Autodesk Inventor part; units mm, degrees
ref_plane "YZ Plane" through (0, 0, 0) normal (1, 0, 0) x (0, 1, 0)
ref_plane "XZ Plane" through (0, 0, 0) normal (0, 1, 0) x (-1, 0, 0)
ref_plane "XY Plane" through (0, 0, 0) normal (0, 0, 1) x (1, 0, 0)
sketch "Sketch1" plane through (0, 0, 0) normal (0, 0, 1) x (1, 0, 0)
  circle A0 centre (0, 0) radius 4.05
  circle A1 centre (0, 0) radius 7.4
  line L0 (-8.7062, 0.25) -> (-2.7169, 0.25)
  line L1 (-2.7169, -0.25) -> (-8.7062, -0.25)
  line L2 (-8.7062, 0.25) -> (-8.7062, -0.25)
  line L3 (-2.7169, 0.25) -> (-2.7169, -0.25)
  point P0 (-4.0423, -0.25)
  point P1 (-7.3958, -0.25)
  point P2 (-7.3958, 0.25)
  point P3 (-4.0423, 0.25)
  dimension "d0" = 8.1
  dimension "d1" = 14.8
  dimension "d2" = 0.25
  dimension "d3" = 0.5
extrude "Extrusion1" add sketch "Sketch1" along normal blind 2 contours A0 L0 A1 L1 picked at (6.1755, 0.9009)
properties part number "Arandela Grower M8"
Read the model definition and answer for the solid it produces. Units are mm, in the model's axes. A direction names the side the tool comes from. Coordinates: 2 decimals unless noted, no trailing zeros. Write each loop counter-clockwise with the first axis right and the second up, starting at its lowest first coordinate (ties: lowest second). Pieces come first, ordered by that corner, then holes. Notation, with made-up numbers: (30.25, -38) - (82.25, -38) arc R6 ccw to (82.25, -28) - close; hole circle Ø1 at (-36.75, -14). An arc over 180 degrees is marked (long way). One line per question, with ' | ' between items.
Q1. Find section A-A, the plane x = 0. Write down the section's boundary in (y, z).
Result set:
outline: (-7.4, 0) - (-4.05, 0) - (-4.05, 2) - (-7.4, 2) - close; (4.05, 0) - (7.4, 0) - (7.4, 2) - (4.05, 2) - close
Q2. Find section B-B, the plane y = -3. Write down the section's boundary in (x, z), plus the area to 3 significant figures.
Result set:
outline: (-6.76, 0) - (-2.72, 0) - (-2.72, 2) - (-6.76, 2) - close; (2.72, 0) - (6.76, 0) - (6.76, 2) - (2.72, 2) - close | area: 16.2 mm^2
Q3. This flat-tipped pin is pushed along its axis until it touches: P1, Ø1, axis at x = -5, z = 1, coming from the -Y side. Where does it stop, or does it pass through?
Result set:
P1: y = -5.87
Q4. Find section C-C, the plane z = 1.3. Write down the section's boundary in (x, y).
Result set:
outline: (-7.4, -0.25) arc R7.4 ccw (long way) to (-7.4, 0.25) - (-4.04, 0.25) arc R4.05 cw (long way) to (-4.04, -0.25) - close
Q5. For faces 1 (the flat face through (-6, -0.25, 1)), 2 (the flat face through (3, -3, 0)), determine the directions among +Z, -Z, +X, -X, +Y, -Y from which every point of the face is accessible in a straight line to the end or side of a thin tool.
Result set:
face 1: +Z, -Z, -X | face 2: -Z, +X, -X, +Y, -Y
Q6. Consider L1, parallel to Y at x = 0, z = 0.8; L2, parallel to Y at x = -5.25, z = 0.8; L3, parallel to X at y = -1.5, z = 0.3. Determine where each line is inside the solid, lowest interval first. Write a range as [from, to].
Result set:
L1: [-7.4, -4.05], [4.05, 7.4] | L2: [-5.22, -0.25], [0.25, 5.22] | L3: [-7.25, -3.76], [3.76, 7.25]
